Geometry: final body of the model. Coordinates: model frame, mm. Give positions to 0.01 mm unless a question says otherwise; leave off trailing zeros. Order: outer loops, then holes, each group sorted by start corner. A loop starts at its lowest first (then second) coordinate and runs counter-clockwise, first axis right, second up. Notation, with made-up numbers: M 82,45.5 L 135,45.5 A13 ccw 135,56.5 Z; hole C 33.25,61 d11. An arc over 180 degrees is marked long. Use CSV: the item, a comma, the result in double quotes.
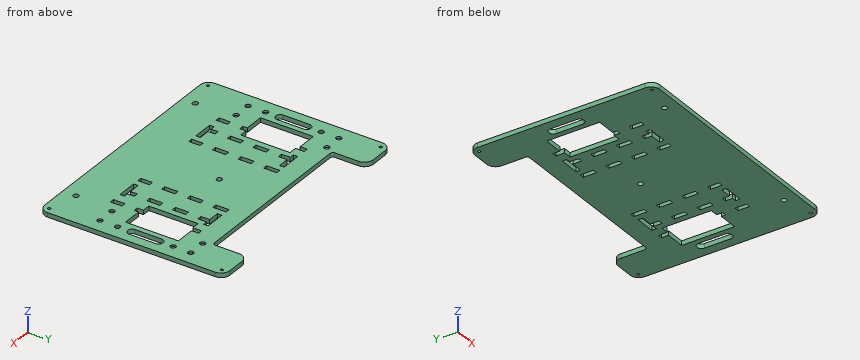
```python
from build123d import *

# Parameters (mm, degrees)
BOSS_EXTRU_1_DEPTH      = 5
ESQUISSE2_W             = 5.07
ESQUISSE2_H             = 13
ESQUISSE2_H_2           = 15
ENL_V_MAT_EXTRU_1_DEPTH = 10
ESQUISSE3_R             = 3.05
ENL_V_MAT_EXTRU_2_DEPTH = 2
ENL_V_MAT_EXTRU_3_DEPTH = 176.071414
ESQUISSE5_R             = 3.05
ESQUISSE5_R_2           = 1.55
ENL_V_MAT_EXTRU_4_DEPTH = 176.071414


with BuildPart() as part:
    # Esquisse1 → Boss.-Extru.1 (new body)
    with BuildSketch(Plane.XY):
        with BuildLine():
            Line((130, -105), (-130, -105))
            ThreePointArc((-130, -105), (-137.071067812, -102.071067812), (-140, -95))
            Line((-140, -95), (-140, 105))
            Line((-140, 105), (140, 105))
            Line((140, 105), (140, -95))
            ThreePointArc((140, -95), (137.071067812, -102.071067812), (130, -105))
        make_face()
    extrude(amount=BOSS_EXTRU_1_DEPTH)

    # Esquisse2 → Enlèv. mat.-Extru.1 (cut)
    with BuildSketch(Plane.XY.offset(5)):
        Polygon((-91, 35), (-113, 35), (-113, -25), (-91, -25), (-91, -30), (-85.93, -30), (-85.93, -23), (-76.93, -23), (-76.93, 33), (-85.93, 33), (-85.93, 43), (-91, 43), align=None)
        with Locations((-88.465, -50.5)):
            Rectangle(ESQUISSE2_W, ESQUISSE2_H)
        with Locations((-67.465, 6.5)):
            Rectangle(ESQUISSE2_W, ESQUISSE2_H_2)
        Polygon((-70, 28), (-64.93, 28), (-64.93, 37.93), (-52, 37.93), (-52, 43), (-75.07, 43), (-75.07, 37.93), (-70, 37.93), align=None)
        Polygon((-52, -57), (-52, -51.93), (-64.93, -51.93), (-64.93, -44), (-70, -44), (-70, -51.93), (-75.07, -51.93), (-75.07, -57), align=None)
        with Locations((-67.465, -22.5)):
            Rectangle(ESQUISSE2_W, ESQUISSE2_H_2)
        with Locations((-42.465, 6.5)):
            Rectangle(ESQUISSE2_W, ESQUISSE2_H_2)
        with Locations((-42.465, 35.5)):
            Rectangle(ESQUISSE2_W, ESQUISSE2_H_2)
        with Locations((-42.465, -50.5)):
            Rectangle(ESQUISSE2_W, ESQUISSE2_H)
        with Locations((-42.465, -22.5)):
            Rectangle(ESQUISSE2_W, ESQUISSE2_H_2)
        Polygon((52, -51.93), (52, -57), (75.07, -57), (75.07, -51.93), (70, -51.93), (70, -44), (64.93, -44), (64.93, -51.93), align=None)
        Polygon((52, 43), (52, 37.93), (64.93, 37.93), (64.93, 28), (70, 28), (70, 37.93), (75.07, 37.93), (75.07, 43), align=None)
        with Locations((42.465, -50.5)):
            Rectangle(ESQUISSE2_W, ESQUISSE2_H)
        with Locations((42.465, -22.5)):
            Rectangle(ESQUISSE2_W, ESQUISSE2_H_2)
        with Locations((42.465, 6.5)):
            Rectangle(ESQUISSE2_W, ESQUISSE2_H_2)
        with Locations((42.465, 35.5)):
            Rectangle(ESQUISSE2_W, ESQUISSE2_H_2)
        with Locations((67.465, -22.5)):
            Rectangle(ESQUISSE2_W, ESQUISSE2_H_2)
        with Locations((67.465, 6.5)):
            Rectangle(ESQUISSE2_W, ESQUISSE2_H_2)
        with Locations((88.465, -50.5)):
            Rectangle(ESQUISSE2_W, ESQUISSE2_H)
        Polygon((85.93, -30), (91, -30), (91, -25), (113, -25), (113, 35), (91, 35), (91, 43), (85.93, 43), (85.93, 33), (76.93, 33), (76.93, -23), (85.93, -23), align=None)
    extrude(amount=-ENL_V_MAT_EXTRU_1_DEPTH, mode=Mode.SUBTRACT)

    # Esquisse3 → Enlèv. mat.-Extru.2 (cut)
    with BuildSketch(Plane.XY.offset(5)):
        with Locations((-124, -26.5)):
            Circle(ESQUISSE3_R)
        with Locations((-124, 36.5)):
            Circle(ESQUISSE3_R)
        with Locations(Location((124, 36.5, 0), (0, 0, 180))):
            Circle(ESQUISSE3_R)
        with Locations(Location((124, -26.5, 0), (0, 0, 180))):
            Circle(ESQUISSE3_R)
        with Locations((-124, 56.5)):
            Circle(ESQUISSE3_R)
        with Locations((-104, 56.5)):
            Circle(ESQUISSE3_R)
        with Locations(Location((-104, -46.5, 0), (0, 0, 180))):
            Circle(ESQUISSE3_R)
        with Locations(Location((-124, -46.5, 0), (0, 0, 180))):
            Circle(ESQUISSE3_R)
        with Locations((124, -46.5)):
            Circle(ESQUISSE3_R)
        with Locations((104, -46.5)):
            Circle(ESQUISSE3_R)
        with Locations(Location((104, 56.5, 0), (0, 0, 180))):
            Circle(ESQUISSE3_R)
        with Locations(Location((124, 56.5, 0), (0, 0, 180))):
            Circle(ESQUISSE3_R)
    extrude(amount=-ENL_V_MAT_EXTRU_2_DEPTH, mode=Mode.SUBTRACT)

    # Esquisse4 → Enlèv. mat.-Extru.3 (cut, through all)
    with BuildSketch(Plane.XY.offset(5)):
        with BuildLine():
            Line((-119, 20), (-119, -10))
            ThreePointArc((-119, -10), (-124, -15), (-129, -10))
            Line((-129, -10), (-129, 20))
            ThreePointArc((-129, 20), (-124, 25), (-119, 20))
        make_face()
        with BuildLine():
            Line((119, 20), (119, -10))
            ThreePointArc((119, -10), (124, -15), (129, -10))
            Line((129, -10), (129, 20))
            ThreePointArc((129, 20), (124, 25), (119, 20))
        make_face()
        with BuildLine():
            Line((-110, 105), (110, 105))
            ThreePointArc((110, 105), (102.928932188, 102.071067812), (100, 95))
            Line((100, 95), (100, 68))
            ThreePointArc((100, 68), (99.121320344, 65.878679656), (97, 65))
            Line((97, 65), (-97, 65))
            ThreePointArc((-97, 65), (-99.121320344, 65.878679656), (-100, 68))
            Line((-100, 68), (-100, 95))
            ThreePointArc((-100, 95), (-102.928932188, 102.071067812), (-110, 105))
        make_face()
        with BuildLine():
            Line((140, 105), (130, 105))
            ThreePointArc((130, 105), (137.071067812, 102.071067812), (140, 95))
            Line((140, 95), (140, 105))
        make_face()
        with BuildLine():
            Line((-140, 95), (-140, 105))
            Line((-140, 105), (-130, 105))
            ThreePointArc((-130, 105), (-137.071067812, 102.071067812), (-140, 95))
        make_face()
    extrude(amount=-ENL_V_MAT_EXTRU_3_DEPTH, mode=Mode.SUBTRACT)

    # Esquisse5 → Enlèv. mat.-Extru.4 (cut, through all)
    with BuildSketch(Plane.XY.offset(5)):
        with Locations((0, 5)):
            Circle(ESQUISSE5_R)
        with Locations((-133, 98)):
            Circle(ESQUISSE5_R_2)
        with Locations((-100, -90)):
            Circle(ESQUISSE5_R)
        with Locations((-133, -98)):
            Circle(ESQUISSE5_R_2)
        with Locations((133, -98)):
            Circle(ESQUISSE5_R_2)
        with Locations((100, -90)):
            Circle(ESQUISSE5_R)
        with Locations((133, 98)):
            Circle(ESQUISSE5_R_2)
    extrude(amount=-ENL_V_MAT_EXTRU_4_DEPTH, mode=Mode.SUBTRACT)


solid = part.part
```
1. Section A-A, the plane x = 124. Return the cut outline in (y, z), plus the area to 3 significant figures.
Answer:
outline,"M -105,0 L -15,0 L -15,5 L -23.45,5 L -23.45,3 L -29.55,3 L -29.55,5 L -43.45,5 L -43.45,3 L -49.55,3 L -49.55,5 L -105,5 Z; M 25,0 L 105,0 L 105,5 L 59.55,5 L 59.55,3 L 53.45,3 L 53.45,5 L 39.55,5 L 39.55,3 L 33.45,3 L 33.45,5 L 25,5 Z"
area,"801 mm2"
2. Section C-C, the plane x = 9.5. Return the cut outline in (y, z).
Answer:
outline,"M -105,0 L 65,0 L 65,5 L -105,5 Z"
3. Line query: line 1 (Y direction, x = -104, z = 4.65); line 2 (Y direction, x = -64, z = 3.35); line 3 (Y direction, x = 65, z = 0.35). Output: solid intervals per line, ascending.
Answer:
line 1,"-105 to -49.55, -43.45 to -25, 35 to 53.45, 59.55 to 103"
line 2,"-105 to -57, -51.93 to 37.93, 43 to 65"
line 3,"-105 to -57, -44 to -30, -15 to -1, 14 to 28, 43 to 65"
4. Section B-B, the plane z = 1.25. Give the number of separate pieces and of enclosed holes in the cut face, plus the area to 3 significant figures.
Answer:
separate pieces,"1"
enclosed holes,"29"
area,"43,700 mm2"
5. Pin query (flat end, axial travel): pin 1 Ø2.5 at (x, z) = (41.5, 3.5) entering from +Y. Return the tip coordinate at first contact, or that it passes through.
Answer:
pin 1,"y = 65"
